Can you work these out from the drawing? Everything is in mm from the part's minimum corner. Give positions to 0.01 mm unless a question says otherwise; leave off trailing zeros. Loops run counter-clockwise (first coordinate to the right, second up) from the corner with the lowest first, then second, coordinate; pieces in that order, holes last. Notation, with made-up numbers: (0, 28.5) - (26, 28.5) arc R22 ccw to (26, 40.5) - close; hole circle Ø8 at (-27, 32.5). An arc over 180 degrees is marked (long way). Answer in a Markdown table with one row per item.
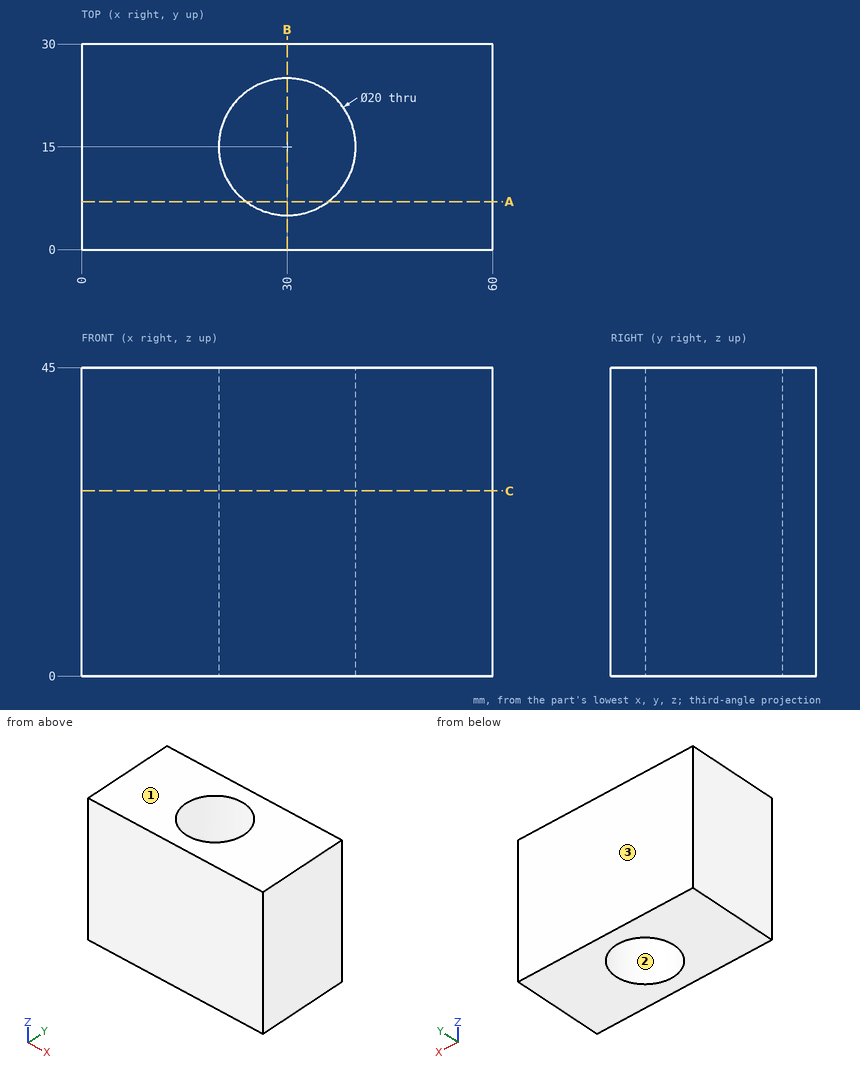
Q1. Imagine slicing it at A-A, the plane y = 7. Write out the boundary of the cut face in (x, z), and give its area (3 significant figures).
Checked values:
| item | result |
|---|---|
| outline | (0, 0) - (24, 0) - (24, 45) - (0, 45) - close; (36, 0) - (60, 0) - (60, 45) - (36, 45) - close |
| area | 2,160 mm² |
Q2. Imagine slicing it at C-C, the plane z = 27. Write out the boundary of the cut face in (x, y), and give its area (3 significant figures).
Checked values:
| item | result |
|---|---|
| outline | (0, 0) - (60, 0) - (60, 30) - (0, 30) - close; hole circle Ø20 at (30, 15) |
| area | 1,490 mm² |
Q3. If we mould it in two halves opening along Y, with no side actions, what happens to the marked faces 1, 2 and 3? For each: released by +Y, released by -Y, zero draft, split by the parting line, or undercut.
Checked values:
| item | result |
|---|---|
| face 1 | zero draft |
| face 2 | undercut |
| face 3 | released by +Y |
Q4. Imagine slicing it at B-B, the plane x = 30. Write out the boundary of the cut face in (y, z).
Checked values:
| item | result |
|---|---|
| outline | (0, 0) - (5, 0) - (5, 45) - (0, 45) - close; (25, 0) - (30, 0) - (30, 45) - (25, 45) - close |
Q5. If I drill on line 1 (Y direction, x = 30, z = 27); line 2 (X direction, y = 9.25, z = 18); line 3 (X direction, y = 20.25, z = 11.5), over which ranges is the centre line in solid material (lowest first)? Write a range as [from, to].
Checked values:
| item | result |
|---|---|
| line 1 | y = [0, 5], [25, 30] |
| line 2 | x = [0, 21.82], [38.18, 60] |
| line 3 | x = [0, 21.49], [38.51, 60] |
